Geometry check sheet. Reference: the model listing, model coordinates, mm. Round coordinates to 2 decimals unless told otherwise and drop trailing zeros. Order: outer loops, then holes, each group sorted by start corner. A loop starts at its lowest first (then second) coordinate and runs counter-clockwise, first axis right, second up. Notation, with made-up numbers: (-11, 84) -> (-6, 84) arc R21 ccw to (-6, 90) -> close; hole circle Ø6 at (5.25, -29). An arc over 180 degrees is marked (long way). Answer as a JSON object with one key per item and string values. Group by question number.
from build123d import *

# Parameters (mm, degrees)
F0_R            = 24.51608
F0_R_2          = 2.15265
F0_R_3          = 7.9375
F1_DEPTH        = 5.08
F3_DEPTH        = 5.08
F3_COPIES_COUNT = 4
F4_R            = 0.762


# Not quite as in the source:
# - a pattern or mirror of a feature is missing from the dataset's text; its kind, count and spacing are read off the source's solid


with BuildPart() as f1:
    # F0 (on Top) → F1 (new body)
    with BuildSketch(Plane.XY):
        Circle(F0_R)
        with Locations((-11.7865906, -11.7865906)):
            Circle(F0_R_2, mode=Mode.SUBTRACT)
        with Locations((11.7865906, -11.7865906)):
            Circle(F0_R_2, mode=Mode.SUBTRACT)
        with Locations((-11.7865906, 11.7865906)):
            Circle(F0_R_2, mode=Mode.SUBTRACT)
        Circle(F0_R_3, mode=Mode.SUBTRACT)
        with Locations((11.7865906, 11.7865906)):
            Circle(F0_R_2, mode=Mode.SUBTRACT)
    extrude(amount=F1_DEPTH)

    # F2 (on face) → F3 (cut, through all)
    with BuildSketch(Plane.XY.offset(5.08)):
        with BuildLine():
            ThreePointArc((-12.5005198818, 17.2967828873), (-7.4612395718, 15.2741760893), (-6.553034663, 9.9206307084))
            Line((-6.553034663, 9.9206307084), (-5.9913991959, 9.3589952413))
            ThreePointArc((-5.9913991959, 9.3589952413), (0, 11.1125), (5.9913991959, 9.3589952413))
            Line((5.9913991959, 9.3589952413), (6.553034663, 9.9206307084))
            ThreePointArc((6.553034663, 9.9206307084), (7.4612395718, 15.2741760893), (12.5005198818, 17.2967828873))
            ThreePointArc((12.5005198818, 17.2967828873), (0, 21.34108), (-12.5005198818, 17.2967828873))
        make_face()
    f3 = extrude(amount=-F3_DEPTH, mode=Mode.SUBTRACT)

    # F3_copies: F3 ×4 about axis
    f3_copies_axis = Axis((0, 0, 0), (0, 0, 1))
    for i in range(1, F3_COPIES_COUNT):
        add(f3.rotate(f3_copies_axis, i * 360 / F3_COPIES_COUNT), mode=Mode.SUBTRACT)

    # F4
    f4_edges = [f1.edges().sort_by_distance(p)[0] for p in [
        (-12.50052, 17.296783, 2.54),
        (12.50052, 17.296783, 2.54),
        (-17.296783, -12.50052, 2.54),
        (-17.296783, 12.50052, 2.54),
        (12.50052, -17.296783, 2.54),
        (-12.50052, -17.296783, 2.54),
        (17.296783, 12.50052, 2.54),
        (17.296783, -12.50052, 2.54),
    ]]
    fillet(f4_edges, radius=F4_R)


solid = f1.part
Item 1: Thickness scan on L1, parallel to X at y = 2, z = 3.05; L2, parallel to Y at x = 5, z = 2.7; L3, parallel to Y at x = -13, z = 2.2. Record the ranges inside material, lowest first.
Item 2: Mould release check, pull along Y, two halves, no side actions. Record for faces 1 (the cylindrical face through (-3.192, 24.307, 2.504)), 2 (the flat face through (10.6, 0.3, 5.08)), 3 (the cylindrical face through (-21.34, 0.15, 2.58)): pulls with the +Y half, pulls with the -Y half, needs draft (parallel to the pull), parting line crosses it, or undercut.
Item 3: Sectioned sample at C-C, the plane y = 19.5. Enter the section's corners in (x, z).
Item 4: Sectioned sample at D-D, the plane z = 3.6. Count the separate pieces of the cut face and the enclosed holes in it, then the cut area to 3 significant figures.
Item 5: Sectioned sample at A-A, the plane y = 0. Enter the section's corners in (x, z).
Item 6: Depth check by flat-ended pin: pin 1 Ø3 at (x, z) = (4.5, 1) entering from +Y; pin 2 Ø1 at (x, z) = (-16.5, 2) entering from +Y; pin 3 Ø1 at (x, z) = (19, 1) entering from -Y. Enter the tip coordinate at first touch or a pass-through.
Result:
{
 "1": {"L1": "x = -24.43 to -21.25, -10.93 to -7.68, 7.68 to 10.93, 21.25 to 24.43", "L2": "y = -24 to -20.75, -9.92 to -6.16, 6.16 to 9.92, 20.75 to 24", "L3": "y = -20.79 to -13.56, -10.01 to -6.36, 6.36 to 10.01, 13.56 to 20.79"},
 "2": {"face 1": "parting line crosses it", "face 2": "needs draft", "face 3": "undercut"},
 "3": {"outline": "(-14.86, 0) -> (-8.67, 0) -> (-8.67, 5.08) -> (-14.86, 5.08) -> close; (8.67, 0) -> (14.86, 0) -> (14.86, 5.08) -> (8.67, 5.08) -> close"},
 "4": {"separate pieces": "1", "enclosed holes": "9", "area": "973 mm2"},
 "5": {"outline": "(-24.52, 0) -> (-21.34, 0) -> (-21.34, 5.08) -> (-24.52, 5.08) -> close; (-11.11, 0) -> (-7.94, 0) -> (-7.94, 5.08) -> (-11.11, 5.08) -> close; (7.94, 0) -> (11.11, 0) -> (11.11, 5.08) -> (7.94, 5.08) -> close; (21.34, 0) -> (24.52, 0) -> (24.52, 5.08) -> (21.34, 5.08) -> close"},
 "6": {"pin 1": "stops at y = 24.33", "pin 2": "stops at y = 18.58", "pin 3": "stops at y = -16.09"}
}
